Geometry: final body of the model. Coordinates: model frame, mm. A direction names the side the tool comes from. Give positions to 0.01 mm unless a question says otherwise; leave off trailing zeros. Loops run counter-clockwise (first coordinate to the right, second up) from the corner with the lowest first, then second, coordinate; pieces in that order, holes last. Notation, with made-up numbers: (-17, 19.5) - (38, 19.5) arc R21 cw to (38, 28.5) - close; hole circle Ø5 at (86.25, 46.5). An arc over 180 degrees is marked (long way). Use CSV: the item, a comma, the result in double quotes. Start each with the question number.
```python
from build123d import *

# Parameters (mm, degrees)
BOSS_EXTRUDE1_DEPTH           = 0.5
SKETCH2_R                     = 0.5
BOSS_EXTRUDE2_DEPTH           = 2
BOSS_EXTRUDE2_DRAFT           = 5
BOSS_EXTRUDE2_PROFILE_2_DEPTH = 2
BOSS_EXTRUDE2_PROFILE_2_DRAFT = 5
BOSS_EXTRUDE2_PROFILE_3_DEPTH = 2
BOSS_EXTRUDE2_PROFILE_3_DRAFT = 5
BOSS_EXTRUDE2_PROFILE_4_DEPTH = 2
BOSS_EXTRUDE2_PROFILE_4_DRAFT = 5
BOSS_EXTRUDE3_REACH           = 25.637
BOSS_EXTRUDE3_END_RADIUS      = 8.5
SKETCH5_RX                    = 3
SKETCH5_RY                    = 1.15


with BuildPart() as part:
    # Sketch1 → Boss-Extrude1 (new, symmetric)
    with BuildSketch(Plane.XY):
        with BuildLine():
            Line((-8.261355821, 2), (-18.261355821, 2))
            Line((-18.261355821, 2), (-18.261355821, -2))
            Line((-18.261355821, -2), (-8.261355821, -2))
            ThreePointArc((-8.261355821, -2), (-8.5, 0), (-8.261355821, 2))
        make_face()
        with BuildLine():
            Line((-5.94e-07, 8.5), (-5.94e-07, 6.5))
            ThreePointArc((-5.94e-07, 6.5), (-6.5, 0), (-5.94e-07, -6.5))
            Line((-5.94e-07, -6.5), (-5.94e-07, -8.5))
            ThreePointArc((-5.94e-07, -8.5), (-8.5, 0), (-5.94e-07, 8.5))
        make_face()
        with BuildLine():
            ThreePointArc((-5.94e-07, 8.5), (-0.626706342, 8.476864937), (-1.250000594, 8.407585772))
            Line((-1.250000594, 8.407585772), (-1.250000594, 6.5))
            Line((-1.250000594, 6.5), (-5.94e-07, 6.5))
            Line((-5.94e-07, 6.5), (-5.94e-07, 8.5))
        make_face()
        with BuildLine():
            Line((-1.250000594, -6.5), (-1.250000594, -8.407585772))
            ThreePointArc((-1.250000594, -8.407585772), (-0.626706342, -8.476864937), (-5.94e-07, -8.5))
            Line((-5.94e-07, -8.5), (-5.94e-07, -6.5))
            Line((-5.94e-07, -6.5), (-1.250000594, -6.5))
        make_face()
    extrude(amount=BOSS_EXTRUDE1_DEPTH, both=True)


with BuildPart() as boss_extrude2_tool:
    # Sketch2 → Boss-Extrude2 (with draft: the straight prism first)
    with BuildSketch(Plane(origin=(0, 2, 0), x_dir=(1, 0, 0), z_dir=(0, 1, 0))):
        with Locations((-17.261355821, 0)):
            Circle(SKETCH2_R)
    extrude(amount=BOSS_EXTRUDE2_DEPTH)
    # Boss-Extrude2: the draft: its side faces are tilted about the plane it starts from
    boss_extrude2_sides = [boss_extrude2_tool.faces().sort_by_distance(p)[0] for p in [
        (-17.761355821, 3, 0),
    ]]
    draft(boss_extrude2_sides, Plane(origin=(0, 2, 0), x_dir=(1, 0, 0), z_dir=(0, 1, 0)), BOSS_EXTRUDE2_DRAFT)


with BuildPart() as part_1:
    add(part.part)

    # Boss-Extrude2: add boss_extrude2_tool
    add(boss_extrude2_tool.part)


with BuildPart() as boss_extrude2_profile_2_tool:
    # Sketch2 → Boss-Extrude2 profile 2 (with draft: the straight prism first)
    with BuildSketch(Plane(origin=(0, 2, 0), x_dir=(1, 0, 0), z_dir=(0, 1, 0))):
        with Locations((-15.161355821, 0)):
            Circle(SKETCH2_R)
    extrude(amount=BOSS_EXTRUDE2_PROFILE_2_DEPTH)
    # Boss-Extrude2 profile 2: the draft: its side faces are tilted about the plane it starts from
    boss_extrude2_profile_2_sides = [boss_extrude2_profile_2_tool.faces().sort_by_distance(p)[0] for p in [
        (-15.661355821, 3, 0),
    ]]
    draft(boss_extrude2_profile_2_sides, Plane(origin=(0, 2, 0), x_dir=(1, 0, 0), z_dir=(0, 1, 0)), BOSS_EXTRUDE2_PROFILE_2_DRAFT)


with BuildPart() as part_2:
    add(part_1.part)

    # Boss-Extrude2 profile 2: add boss_extrude2_profile_2_tool
    add(boss_extrude2_profile_2_tool.part)


with BuildPart() as boss_extrude2_profile_3_tool:
    # Sketch2 → Boss-Extrude2 profile 3 (with draft: the straight prism first)
    with BuildSketch(Plane(origin=(0, 2, 0), x_dir=(1, 0, 0), z_dir=(0, 1, 0))):
        with Locations((-13.061355821, 0)):
            Circle(SKETCH2_R)
    extrude(amount=BOSS_EXTRUDE2_PROFILE_3_DEPTH)
    # Boss-Extrude2 profile 3: the draft: its side faces are tilted about the plane it starts from
    boss_extrude2_profile_3_sides = [boss_extrude2_profile_3_tool.faces().sort_by_distance(p)[0] for p in [
        (-13.561355821, 3, 0),
    ]]
    draft(boss_extrude2_profile_3_sides, Plane(origin=(0, 2, 0), x_dir=(1, 0, 0), z_dir=(0, 1, 0)), BOSS_EXTRUDE2_PROFILE_3_DRAFT)


with BuildPart() as part_3:
    add(part_2.part)

    # Boss-Extrude2 profile 3: add boss_extrude2_profile_3_tool
    add(boss_extrude2_profile_3_tool.part)


with BuildPart() as boss_extrude2_profile_4_tool:
    # Sketch2 → Boss-Extrude2 profile 4 (with draft: the straight prism first)
    with BuildSketch(Plane(origin=(0, 2, 0), x_dir=(1, 0, 0), z_dir=(0, 1, 0))):
        with Locations((-10.961355821, 0)):
            Circle(SKETCH2_R)
    extrude(amount=BOSS_EXTRUDE2_PROFILE_4_DEPTH)
    # Boss-Extrude2 profile 4: the draft: its side faces are tilted about the plane it starts from
    boss_extrude2_profile_4_sides = [boss_extrude2_profile_4_tool.faces().sort_by_distance(p)[0] for p in [
        (-11.461355821, 3, 0),
    ]]
    draft(boss_extrude2_profile_4_sides, Plane(origin=(0, 2, 0), x_dir=(1, 0, 0), z_dir=(0, 1, 0)), BOSS_EXTRUDE2_PROFILE_4_DRAFT)


with BuildPart() as part_4:
    add(part_3.part)

    # Boss-Extrude2 profile 4: add boss_extrude2_profile_4_tool
    add(boss_extrude2_profile_4_tool.part)

    # Boss-Extrude3: up to this cylinder (the profile starts inside it)
    boss_extrude3_end = Plane(origin=(0, 0, 0), z_dir=(0, 0, -1)) * Cylinder(BOSS_EXTRUDE3_END_RADIUS, 69.274, mode=Mode.PRIVATE)
    # Sketch5 → Boss-Extrude3 (add, up to the surface)
    with BuildSketch(Plane(origin=(0, 6.5, 0), x_dir=(1, 0, 0), z_dir=(0, 1, 0)), mode=Mode.PRIVATE) as boss_extrude3_sk1:
        with Locations((0, 0)):
            Ellipse(SKETCH5_RX, SKETCH5_RY)
    boss_extrude3_tool1 = extrude(boss_extrude3_sk1.sketch, amount=BOSS_EXTRUDE3_REACH, mode=Mode.PRIVATE) & boss_extrude3_end
    boss_extrude3 = boss_extrude3_tool1.solids().sort_by_distance((0, 6.5, 0))[0]
    add(boss_extrude3)

    # Mirror1: Boss-Extrude3 across plane
    add(boss_extrude3.mirror(Plane.ZX))


solid = part_4.part
```
Item 1: Pin query (flat end, axial travel): pin 1 Ø6 at (x, y) = (-11, 1) entering from -Z; pin 2 Ø1 at (y, z) = (-3.5, 0) entering from -X; pin 3 Ø1.5 at (x, y) = (-15.5, 0.5) entering from +Z. Return the tip coordinate at first contact, or that it passes through.
Item 2: Section B-B (y = 0). Output: boundary loops of the cut face in (x, z), plus the area to 3 significant figures.
Item 3: Section A-A (x = -3.25). Output: boundary loops of the cut face in (y, z).
Item 4: Mould query, pull axis Y, two halves, no side actions, for faces 4 (the flat face through (-18.261, 0, 0)), 5 (the flat face through (1, 6.5, 0)), 6 (the flat face through (1, -6.5, 0)), 7 (the flat face through (-9, 2, 0)). Classes: pulls with the +Y half, pulls with the -Y half, needs draft (parallel to the pull), parting line crosses it, or undercut.
Item 5: Reachability of faces 1 (the flat face through (-18, 2, 0)), 2 (the conical face through (-12.84, 2.99, -0.35)), 3 (the flat face through (-13, -2, 0)) from +Z, -Z, +X, -X, +Y, -Y: full face, straight path, thin tool, end or side. Return the list, or none.
Item 6: Section C-C (x = -9.75). Output: boundary loops of the cut face in (y, z), plus the area to 3 significant figures.
Item 7: Ray query, probe 1 along Y at (x, z) = (-2, 0.6); probe 2 along Z at (x, y) = (-15.5, 1.5); probe 3 along Y at (x, z) = (-14.5, 0). Return the intervals inside material, ascending.
Outcome:
1,pin 1,"stops at z = -0.5"
1,pin 2,"stops at x = -7.95"
1,pin 3,"stops at z = 0.5"
2,outline,"(-18.26, -0.5) - (-6.5, -0.5) - (-6.5, 0.5) - (-18.26, 0.5) - close"
2,area,"11.8 mm2"
3,outline,"(-7.85, -0.5) - (-5.63, -0.5) - (-5.63, 0.5) - (-7.85, 0.5) - close; (5.63, -0.5) - (7.85, -0.5) - (7.85, 0.5) - (5.63, 0.5) - close"
4,face 4,"needs draft"
4,face 5,"undercut"
4,face 6,"undercut"
4,face 7,"pulls with the +Y half"
5,face 1,"-X, +Y"
5,face 2,"+Y"
5,face 3,"+Z, -Z, -X, -Y"
6,outline,"(-2, -0.5) - (2, -0.5) - (2, 0.5) - (-2, 0.5) - close"
6,area,"4.00 mm2"
7,probe 1,"y = -8.26 to -6.5, 6.5 to 8.26"
7,probe 2,"z = -0.5 to 0.5"
7,probe 3,"y = -2 to 2"
